from build123d import *

# Parameters (mm, degrees)
SKETCH_W            = 84
SKETCH_H            = 94.6
PAD_DEPTH           = 15
SKETCH001_R         = 9.75
POCKET_DEPTH        = 94.601
LINEARPATTERN_COUNT = 3
LINEARPATTERN_PITCH = 28
HOLE_D              = 5
HOLE_DEPTH          = 25
HOLE_CSINK_D        = 11
HOLE_CSINK_ANGLE    = 90
SKETCH003_R         = 2.8
POCKET001_DEPTH     = 15.001
POCKET002_DEPTH     = 84.001


with BuildPart() as part:
    # Sketch → Pad (new body)
    with BuildSketch(Plane.XY):
        with Locations((42, 47.3)):
            Rectangle(SKETCH_W, SKETCH_H)
    extrude(amount=PAD_DEPTH)

    # Sketch001 (on DatumPlane) → Pocket (cut, through all)
    with BuildSketch(Plane.XZ):
        with Locations((14, 15)):
            Circle(SKETCH001_R)
    pocket = extrude(amount=-POCKET_DEPTH, mode=Mode.SUBTRACT)

    # LinearPattern: Pocket ×3
    with Locations(*[(i * LINEARPATTERN_PITCH, 0, 0) for i in range(1, LINEARPATTERN_COUNT)]):
        add(pocket, mode=Mode.SUBTRACT)

    # Hole
    with Locations(Plane(origin=(0, 0, 0), x_dir=(1, 0, 0), z_dir=(0, 0, -1))):
        with Locations((28, -6), (56, -6), (28, -88.6), (56, -88.6)):
            CounterSinkHole(HOLE_D / 2, HOLE_CSINK_D / 2, depth=HOLE_DEPTH, counter_sink_angle=HOLE_CSINK_ANGLE)

    # Sketch003 → Pocket001 (cut, through all)
    with BuildSketch(Plane.XY):
        with Locations((42, 88.6)):
            Circle(SKETCH003_R)
        with Locations((42, 6)):
            Circle(SKETCH003_R)
    extrude(amount=POCKET001_DEPTH, mode=Mode.SUBTRACT)

    # Sketch004 (on DatumPlane) → Pocket002 (cut, through all)
    with BuildSketch(Plane.YZ):
        Polygon((82.6, 15), (12, 15), (21.75, 5.25), (72.85, 5.25), align=None)
    extrude(amount=POCKET002_DEPTH, mode=Mode.SUBTRACT)


solid = part.part
The model under review builds one solid part; all positions refer to its coordinate system, in mm. A direction names the side the tool comes from. Round coordinates to 2 decimals unless told otherwise and drop trailing zeros. Loops run counter-clockwise (first coordinate to the right, second up) from the corner with the lowest first, then second, coordinate; pieces in that order, holes last. Notation, with made-up numbers: (37, -6.75) -> (47, -6.75) arc R22 cw to (47, 24.25) -> close; hole circle Ø10 at (59.5, 42.5). An arc over 180 degrees is marked (long way). Write item = value, one per line. Start each with the question number.
Item 1: Take a section at A-A on x = 28. Give the boundary of the cut face in (y, z).
Item 2: Mouldability with a two-part tool opening along Y and no side actions: class faces 3 (the flat face through (55.8, 76.6, 9)), 4 (the flat face through (2, 6, 15)) as released by +Y, released by -Y, zero draft, split by the parting line, or undercut.
Item 3: Take a section at C-C on z = 1.5. Give the boundary of the cut face in (x, y), plus the area to 3 significant figures.
Item 4: To check wall thickness, follow L1, parallel to Y at x = 42, z = 4.15; L2, parallel to Y at x = 27.5, z = 3.5; L3, parallel to Y at x = 55.5, z = 5.5. State the ranges of each line that lie inside material, in increasing order.
Item 5: For faces 1 (the flat face through (41, 48, 0)), 2 (the flat face through (3.8, 76.6, 9)), list the 3-axis set-ups (+Z, -Z, +X, -X, +Y, -Y) from which the entire face can be reached by the end or side of a thin tool; tool diameter is ignored.
Item 6: Insertion check: pin 1 (2 mm diameter, centred on x = 51.5, z = 7, fed in from -Y); pin 2 (1 mm diameter, centred on x = 73.5, y = 71, fed in from +Z); pin 3 (7.5 mm diameter, centred on x = 42, y = 88.6, fed in from +Z); pin 4 (9 mm diameter, centred on x = 42, y = 6, fed in from +Z). Each pin has a flat end and moves straight along its axis. Give the tip position at first contact, or say it passes through.
Item 7: Take a section at D-D on y = 18. Give the boundary of the cut face in (x, z).
Item 8: Take a section at B-B on y = 88.6. Give the boundary of the cut face in (x, z).
Result:
q1.outline = (0, 0) -> (0.5, 0) -> (3.5, 3) -> (3.5, 15) -> (0, 15) -> close; (8.5, 3) -> (11.5, 0) -> (83.1, 0) -> (86.1, 3) -> (86.1, 15) -> (82.6, 15) -> (72.85, 5.25) -> (21.75, 5.25) -> (12, 15) -> (8.5, 15) -> close; (91.1, 3) -> (94.1, 0) -> (94.6, 0) -> (94.6, 15) -> (91.1, 15) -> close
q2.face_3 = undercut
q2.face_4 = zero draft
q3.outline = (0, 0) -> (84, 0) -> (84, 94.6) -> (0, 94.6) -> close; hole circle Ø8 at (28, 6); hole circle Ø8 at (28, 88.6); hole circle Ø5.6 at (42, 6); hole circle Ø5.6 at (42, 88.6); hole circle Ø8 at (56, 6); hole circle Ø8 at (56, 88.6)
q3.area = 7,700 mm²
q4.L1 = 0 to 3.2, 8.8 to 85.8, 91.4 to 94.6
q4.L2 = 0 to 3.55, 8.45 to 86.15, 91.05 to 94.6
q4.L3 = 0 to 3.55, 8.45 to 21.5, 73.1 to 86.15, 91.05 to 94.6
q5.face_1 = -Z, +X, -X, +Y, -Y
q5.face_2 = +Z, +X, -X
q6.pin_1 = 0
q6.pin_2 = 5.25
q6.pin_3 = 6
q6.pin_4 = 6.35
q7.outline = (0, 0) -> (84, 0) -> (84, 9) -> (77.69, 9) arc R9.75 cw to (62.31, 9) -> (49.69, 9) arc R9.75 cw to (34.31, 9) -> (21.69, 9) arc R9.75 cw to (6.31, 9) -> (0, 9) -> close
q8.outline = (0, 0) -> (22.5, 0) -> (25.5, 3) -> (25.5, 15) -> (23.75, 15) arc R9.75 cw to (4.25, 15) -> (0, 15) -> close; (30.5, 3) -> (33.5, 0) -> (39.2, 0) -> (39.2, 5.66) arc R9.75 cw to (32.25, 15) -> (30.5, 15) -> close; (44.8, 0) -> (50.5, 0) -> (53.5, 3) -> (53.5, 15) -> (51.75, 15) arc R9.75 cw to (44.8, 5.66) -> close; (58.5, 3) -> (61.5, 0) -> (84, 0) -> (84, 15) -> (79.75, 15) arc R9.75 cw to (60.25, 15) -> (58.5, 15) -> close
